```python
from build123d import *

# Parameters (mm, degrees)
F0_R     = 22.5
F0_R_2   = 10
F1_DEPTH = 3
F2_D     = 3.3
F3_D     = 4.4
F4_R     = 12.6
F4_R_2   = 10
F5_DEPTH = 2
F6_D     = 2.5


with BuildPart() as f1:
    # F0 (on Front) → F1 (new body)
    with BuildSketch(Plane.XZ):
        Circle(F0_R)
        Circle(F0_R_2, mode=Mode.SUBTRACT)
    extrude(amount=F1_DEPTH)

    # F2 (through all)
    with Locations(Plane(origin=(0, 0, 0), x_dir=(1, 0, 0), z_dir=(0, 1, 0))):
        with Locations((-16.4450556787, -6.8117650961), (-6.8117650961, -16.4450556787), (6.8117650961, -16.4450556787), (16.4450556787, -6.8117650961), (16.4450556787, 6.8117650961), (6.8117650961, 16.4450556787), (-6.8117650961, 16.4450556787), (-16.4450556787, 6.8117650961)):
            Hole(F2_D / 2)

    # F3 (through all)
    with Locations(Plane(origin=(0, 0, 0), x_dir=(1, 0, 0), z_dir=(0, 1, 0))):
        with Locations((-17.8, 0), (17.8, 0)):
            Hole(F3_D / 2)

    # F4 (on face) → F5 (cut)
    with BuildSketch(Plane(origin=(0, 0, 0), x_dir=(-1, 0, 0), z_dir=(0, 1, 0))):
        Circle(F4_R)
        Circle(F4_R_2, mode=Mode.SUBTRACT)
    extrude(amount=-F5_DEPTH, mode=Mode.SUBTRACT)

    # F6 (through all)
    with Locations(Plane(origin=(0, 0, 0), x_dir=(1, 0, 0), z_dir=(0, 1, 0))):
        with Locations((0, -17.8), (0, 17.8)):
            Hole(F6_D / 2)


solid = f1.part
```
Geometry check sheet. Reference: the model listing, model coordinates, mm. A direction names the side the tool comes from. Coordinates: 2 decimals unless noted, no trailing zeros. Order: outer loops, then holes, each group sorted by start corner. A loop starts at its lowest first (then second) coordinate and runs counter-clockwise, first axis right, second up.
Q1. Thickness scan on probe 1 along Z at (x, y) = (0, -1.5); probe 2 along Z at (x, y) = (17.5, -0.7); probe 3 along X at (y, z) = (-1.05, -15.5). Record the ranges inside material, lowest first.
Reply:
probe 1: z = -22.5 to -19.05, -16.55 to -12.6, 12.6 to 16.55, 19.05 to 22.5
probe 2: z = -14.14 to -8.08, -5.54 to -2.18, 2.18 to 5.54, 8.08 to 14.14
probe 3: x = -16.31 to -8.16, -5.46 to 5.46, 8.16 to 16.31
Q2. Sectioned sample at A-A on x = 0. Record the cut outline in (y, z).
Reply:
outline: (-3, -22.5) - (0, -22.5) - (0, -19.05) - (-3, -19.05) - close; (-3, -16.55) - (0, -16.55) - (0, -12.6) - (-2, -12.6) - (-2, -10) - (-3, -10) - close; (-3, 10) - (-2, 10) - (-2, 12.6) - (0, 12.6) - (0, 16.55) - (-3, 16.55) - close; (-3, 19.05) - (0, 19.05) - (0, 22.5) - (-3, 22.5) - close
Q3. Draft check along X on faces 3 (the face through (-10.3, -3, 0.3)), 4 (the face through (16.617, -1.521, -1.855)), 5 (the face through (10.382, -1.479, -19.961)). Enter one of: released by +X, released by -X, zero draft, split by the parting line, or undercut.
Reply:
face 3: zero draft
face 4: undercut
face 5: split by the parting line
Q4. Sectioned sample at C-C on y = -0.5. Give the number of separate pieces and of enclosed holes in the cut face, and give its area (3 significant figures).
Reply:
separate pieces: 1
enclosed holes: 13
area: 983 mm2
Q5. Depth check by flat-ended pin: pin 1 Ø2 at (x, z) = (0, -17.8) entering from +Y; pin 2 Ø23 at (x, z) = (0, 0) entering from +Y. Enter the tip coordinate at first touch or a pass-through.
Reply:
pin 1: passes through
pin 2: stops at y = -2
Q6. Sectioned sample at B-B on z = 0. Record the cut outline in (x, y), and give its area (3 significant figures).
Reply:
outline: (-22.5, -3) - (-20, -3) - (-20, 0) - (-22.5, 0) - close; (-15.6, -3) - (-10, -3) - (-10, -2) - (-12.6, -2) - (-12.6, 0) - (-15.6, 0) - close; (10, -3) - (15.6, -3) - (15.6, 0) - (12.6, 0) - (12.6, -2) - (10, -2) - close; (20, -3) - (22.5, -3) - (22.5, 0) - (20, 0) - close
area: 38.2 mm2
Q7. Tool access check on faces 1 (the face through (7.169, -1.521, 18.056)), 2 (the face through (8, -2, 7)). Record the directions out of +Z, -Z, +X, -X, +Y, -Y that give a thin tool (end or side, any length) a straight path to the whole face; none if there is none.
Reply:
face 1: +Y, -Y
face 2: +Y
Q8. Sectioned sample at D-D on z = -12. Record the cut outline in (x, y), and give its area (3 significant figures).
Reply:
outline: (-19.03, -3) - (19.03, -3) - (19.03, 0) - (3.84, 0) - (3.84, -2) - (-3.84, -2) - (-3.84, 0) - (-19.03, 0) - close
area: 98.8 mm2
